Here's how the part is built. I have some questions about the finished solid (model axes, mm). A direction names the side the tool comes from. Round coordinates to 2 decimals unless told otherwise and drop trailing zeros. Write each loop counter-clockwise with the first axis right and the second up, starting at its lowest first coordinate (ties: lowest second). Pieces come first, ordered by that corner, then holes. Notation, with made-up numbers: M -8,46 L 22,46 A35 ccw 22,84 Z; hole C -8.75,-26.5 d9. An arc over 180 degrees is marked long. Use a Markdown table: item, result. Add a question column.
```python
from build123d import *

# Parameters (mm, degrees)
SKETCH1_R           = 1
SKETCH1_R_2         = 2.1
BOSS_EXTRUDE2_DEPTH = 150


with BuildPart() as part:
    # Sketch1 → Boss-Extrude2 (new body)
    with BuildSketch(Plane.XY):
        with BuildLine():
            Line((-6.4, -1.5), (-6.4, -6.65))
            ThreePointArc((-6.4, -6.65), (-6.326776695, -6.826776695), (-6.15, -6.9))
            Line((-6.15, -6.9), (-4.4, -6.9))
            Line((-4.4, -6.9), (-4.4, -4.9))
            Line((-4.4, -4.9), (-2.927777778, -4.9))
            Line((-2.927777778, -4.9), (-0.4, -7.5))
            Line((-0.4, -7.5), (-0.4, -12.5))
            Line((-0.4, -12.5), (-2.927777778, -15.1))
            Line((-2.927777778, -15.1), (-4.4, -15.1))
            Line((-4.4, -15.1), (-4.4, -13.1))
            Line((-4.4, -13.1), (-6.15, -13.1))
            ThreePointArc((-6.15, -13.1), (-6.326776695, -13.173223305), (-6.4, -13.35))
            Line((-6.4, -13.35), (-6.4, -18.5))
            ThreePointArc((-6.4, -18.5), (-5.960660172, -19.560660172), (-4.9, -20))
            Line((-4.9, -20), (0.25, -20))
            ThreePointArc((0.25, -20), (0.426776695, -19.926776695), (0.5, -19.75))
            Line((0.5, -19.75), (0.5, -18))
            Line((0.5, -18), (-1.5, -18))
            Line((-1.5, -18), (-1.5, -16.527777778))
            Line((-1.5, -16.527777778), (1.1, -14))
            Line((1.1, -14), (6.1, -14))
            Line((6.1, -14), (8.7, -16.527777778))
            Line((8.7, -16.527777778), (8.7, -18))
            Line((8.7, -18), (6.7, -18))
            Line((6.7, -18), (6.7, -19.75))
            ThreePointArc((6.7, -19.75), (6.773223305, -19.926776695), (6.95, -20))
            Line((6.95, -20), (12.1, -20))
            ThreePointArc((12.1, -20), (13.160660172, -19.560660172), (13.6, -18.5))
            Line((13.6, -18.5), (13.6, -13.35))
            ThreePointArc((13.6, -13.35), (13.526776695, -13.173223305), (13.35, -13.1))
            Line((13.35, -13.1), (11.6, -13.1))
            Line((11.6, -13.1), (11.6, -15.1))
            Line((11.6, -15.1), (10.127777778, -15.1))
            Line((10.127777778, -15.1), (7.6, -12.5))
            Line((7.6, -12.5), (7.6, -7.5))
            Line((7.6, -7.5), (10.127777778, -4.9))
            Line((10.127777778, -4.9), (11.6, -4.9))
            Line((11.6, -4.9), (11.6, -6.9))
            Line((11.6, -6.9), (13.35, -6.9))
            ThreePointArc((13.35, -6.9), (13.526776695, -6.826776695), (13.6, -6.65))
            Line((13.6, -6.65), (13.6, -1.5))
            ThreePointArc((13.6, -1.5), (13.160660172, -0.439339828), (12.1, 0))
            Line((12.1, 0), (6.95, 0))
            ThreePointArc((6.95, 0), (6.773223305, -0.073223305), (6.7, -0.25))
            Line((6.7, -0.25), (6.7, -2))
            Line((6.7, -2), (8.7, -2))
            Line((8.7, -2), (8.7, -3.472222222))
            Line((8.7, -3.472222222), (6.1, -6))
            Line((6.1, -6), (1.1, -6))
            Line((1.1, -6), (-1.5, -3.472222222))
            Line((-1.5, -3.472222222), (-1.5, -2))
            Line((-1.5, -2), (0.5, -2))
            Line((0.5, -2), (0.5, -0.25))
            ThreePointArc((0.5, -0.25), (0.426776695, -0.073223305), (0.25, 0))
            Line((0.25, 0), (-4.9, 0))
            ThreePointArc((-4.9, 0), (-5.960660172, -0.439339828), (-6.4, -1.5))
        make_face()
        with Locations((-3.95, -2.45)):
            Circle(SKETCH1_R, mode=Mode.SUBTRACT)
        with Locations((11.15, -2.45)):
            Circle(SKETCH1_R, mode=Mode.SUBTRACT)
        with Locations((-3.95, -17.55)):
            Circle(SKETCH1_R, mode=Mode.SUBTRACT)
        with Locations((11.15, -17.55)):
            Circle(SKETCH1_R, mode=Mode.SUBTRACT)
        with Locations((3.6, -10)):
            Circle(SKETCH1_R_2, mode=Mode.SUBTRACT)
    extrude(amount=BOSS_EXTRUDE2_DEPTH)


solid = part.part
```
Item 1: Imagine slicing it at B-B on z = 140. Count the separate pieces of the cut face and the enclosed holes in it, plus the area to 3 significant figures.
Item 2: On a 3-axis mill with a long thin cutter (end or side, diameter ignored), from which of +Z, -Z, +X, -X, +Y, -Y can I reach the whole of each face in a straight line? I mean faces 1 (the face through (4, -14, 74)), 2 (the face through (-0.4, -10, 74)), 3 (the face through (4, -6, 74)), 4 (the face through (7.382, -15.246, 73.95)). Say none if no direction works.
Item 3: For pin 1 Ø0.5 at (x, z) = (-5.5, 72.5) entering from +Y; pin 2 Ø5.5 at (y, z) = (-10, 111.5) entering from +X, each with a flat end and sliding along its axis, tell me the tip position at first contact or that it passes through.
Item 4: Imagine slicing it at A-A on y = -10. List the corners of the cut face in (x, z) for me.
Item 5: I need wall thicknesses on probe 1 along Y at (x, z) = (11.15, 107); probe 2 along Y at (x, z) = (0.25, 96); probe 3 along X at (y, z) = (-6.75, 103.5). Which ranges of each line are inside material? Lowest first, please. Write a range as from..to.
Item 6: If we mould it in two halves opening along X, with no side actions, what happens to faces 5 (the face through (-6.4, -16, 74)), 6 (the face through (-0.218, -15.282, 73.95)), 7 (the face through (-2, -20, 74))? For each: +X half, -X half, draft (parallel to the pull), parting line (faces both ways), or undercut.
The answers:
| question | item | result |
|---|---|---|
| 1 | separate pieces | 1 |
| 1 | enclosed holes | 5 |
| 1 | area | 185 mm² |
| 2 | face 1 | +Z, -Z, -Y |
| 2 | face 2 | +Z, -Z, -X |
| 2 | face 3 | +Z, -Z, +Y |
| 2 | face 4 | +Z, -Z |
| 3 | pin 1 | y = -0.04 |
| 3 | pin 2 | x = 7.84 |
| 4 | outline | M -0.4,0 L 1.5,0 L 1.5,150 L -0.4,150 Z; M 5.7,0 L 7.6,0 L 7.6,150 L 5.7,150 Z |
| 5 | probe 1 | -20..-18.55, -16.55..-15.1, -4.9..-3.45, -1.45..0 |
| 5 | probe 2 | -20..-18, -14.83..-5.17, -2..0 |
| 5 | probe 3 | -6.38..-4.4, -1.13..8.33, 11.6..13.58 |
| 6 | face 5 | -X half |
| 6 | face 6 | undercut |
| 6 | face 7 | draft |
